Study the drawing (mm; zero at the part's minimum x, y, z) and answer. Give positions to 0.01 mm unless a question says otherwise; leave off trailing zeros. Order: outer loops, then holes, each group sorted by start corner. A loop starts at its lowest first (then second) coordinate and runs counter-clockwise, first axis right, second up.
Item 1: A cutting plane is placed at A-A (y = 3.75). Write down the section's boundary in (x, z), plus the area to 3 significant figures.
Item 2: A cutting plane is placed at C-C (x = 0.35). State how many separate pieces and enclosed holes the cut face has, plus the area to 3 significant figures.
Item 3: Find the intervals of material crossed by line 1 along Z through (x, y) = (0.6, 3.75); line 2 along Z through (x, y) = (0.2, 10.25); line 3 along Y through (x, z) = (0.3, 2), in increasing order.
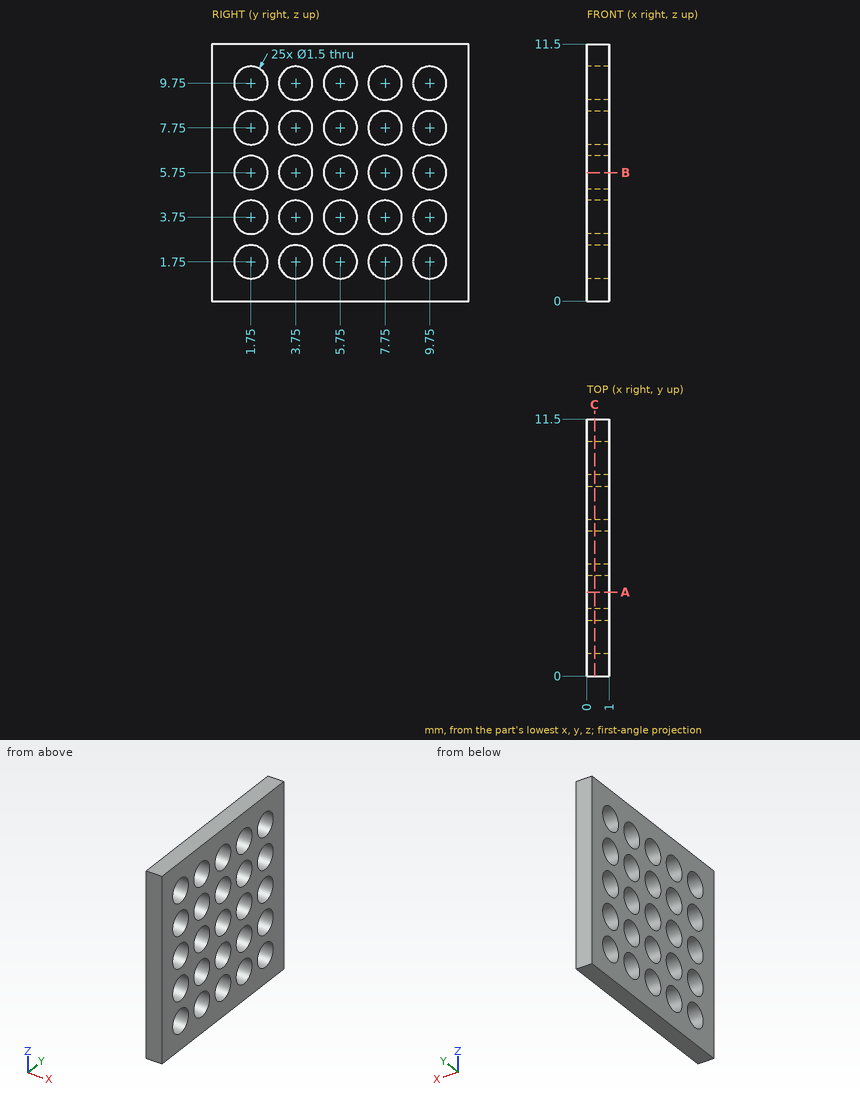
Response values:
1. outline: (0, 0) - (1, 0) - (1, 1) - (0, 1) - close; (0, 2.5) - (1, 2.5) - (1, 3) - (0, 3) - close; (0, 4.5) - (1, 4.5) - (1, 5) - (0, 5) - close; (0, 6.5) - (1, 6.5) - (1, 7) - (0, 7) - close; (0, 8.5) - (1, 8.5) - (1, 9) - (0, 9) - close; (0, 10.5) - (1, 10.5) - (1, 11.5) - (0, 11.5) - close
1. area: 4.00 mm2
2. separate pieces: 1
2. enclosed holes: 25
2. area: 88.1 mm2
3. line 1: z = 0 to 1, 2.5 to 3, 4.5 to 5, 6.5 to 7, 8.5 to 9, 10.5 to 11.5
3. line 2: z = 0 to 1.19, 2.31 to 3.19, 4.31 to 5.19, 6.31 to 7.19, 8.31 to 9.19, 10.31 to 11.5
3. line 3: y = 0 to 1.04, 2.46 to 3.04, 4.46 to 5.04, 6.46 to 7.04, 8.46 to 9.04, 10.46 to 11.5
